```python
from build123d import *

# Parameters (mm, degrees)
F2_R     = 29.7149419412
F0_R     = 50.6662740333
F4_DEPTH = 119.126
F5_T     = -2.54


with BuildPart() as f3:
    # F2 (on offset) → F3 section 0
    with BuildSketch(Plane.XY.offset(49.53)):
        Circle(F2_R)
    # F0 (on Top) → F3 section 1
    with BuildSketch(Plane.XY):
        Circle(F0_R)
    loft()

    # F4 (add): a face of the model
    f4_faces = [f3.faces().sort_by_distance(p)[0] for p in [
        (0, 0, 0),
    ]]
    extrude(f4_faces, amount=F4_DEPTH)

    # F5
    f5_openings = [f3.faces().sort_by_distance(p)[0] for p in [
        (0, 0, 49.53),
    ]]
    offset(amount=F5_T, openings=f5_openings, kind=Kind.INTERSECTION)


solid = f3.part
```
The listing builds one solid part. Answer for the finished solid, in the listing's coordinates (mm). A direction names the side the tool comes from. Give positions to 0.01 mm unless a question says otherwise; leave off trailing zeros. Order: outer loops, then holes, each group sorted by start corner. A loop starts at its lowest first (then second) coordinate and runs counter-clockwise, first axis right, second up. Notation, with made-up numbers: (29.5, -24) - (85.5, -24) arc R12 cw to (85.5, -15) - close; hole circle Ø7 at (8.5, -12). An arc over 180 degrees is marked (long way). Use one line per item in the form item = value. Start each with the question number.
(1) A cutting plane is placed at B-B, the plane x = 0. Write down the section's boundary in (y, z), then the cut area to 3 significant figures.
(2) Flat-ended cylindrical pins translate along their axes: pin 1 Ø12 at (y, z) = (7, -97.5) entering from -X; pin 2 Ø12 at (x, z) = (-26, -100.5) entering from +Y; pin 3 Ø2 at (x, y) = (-36.5, -27) entering from +Z. Find the tip coordinate at first contact, or state that the pin passes through.
(3) A cutting plane is placed at A-A, the plane z = -108. Write down the section's boundary in (x, y).
(4) Consider line 1 (Y direction, x = 0, z = -66); line 2 (Z direction, x = 27, y = 5.5); line 3 (X direction, y = -15.5, z = 23). Determine where each line is inside the solid, lowest interval first. Write a range as from..to.
(5) The mould has two halves that part along Z. Classify faces 3 (the conical face through (-4.34, 33.07, 40.93)), 4 (the cylindrical face through (-10.433, -46.982, -57.738)), 5 (the cylindrical face through (-40.207, -30.83, -58.729)), 6 (the flat face through (-1, 1, -119.126)): released by +Z, released by -Z, zero draft, split by the parting line, or undercut.
(6) A cutting plane is placed at C-C, the plane z = 27.5. Write down the section's boundary in (x, y).
(7) For faces 1 (the flat face through (-6.7, -26.3, 49.53)), 2 (the conical face through (-7.15, -32.2, 35.28)), determine the directions among +Z, -Z, +X, -X, +Y, -Y from which every point of the face is accessible in a straight line to the end or side of a thin tool.
Ans:
q1.outline = (-50.67, -119.13) - (50.67, -119.13) - (50.67, 0) - (29.71, 49.53) - (26.96, 49.53) - (48.13, -0.52) - (48.13, -116.59) - (-48.13, -116.59) - (-48.13, -0.52) - (-26.96, 49.53) - (-29.71, 49.53) - (-50.67, 0) - close
q1.area = 1,120 mm^2
q2.pin_1 = -50.66
q2.pin_2 = 46.55
q2.pin_3 = 14.81
q3.outline = circle Ø101.33 at (0, 0); hole circle Ø96.25 at (0, 0)
q4.line_1 = -50.67..-48.13, 48.13..50.67
q4.line_2 = -119.13..-116.59, 48.12..49.53
q4.line_3 = -37.89..-34.89, 34.89..37.89
q5.face_3 = released by +Z
q5.face_4 = undercut
q5.face_5 = zero draft
q5.face_6 = released by -Z
q6.outline = circle Ø78.07 at (0, 0); hole circle Ø72.55 at (0, 0)
q7.face_1 = +Z, +X, -X, +Y, -Y
q7.face_2 = none
